Print and shaded views of the part. All mm, measured from the part's lowest x, y and z. A direction names the side the tool comes from. Round coordinates to 2 decimals unless told otherwise and drop trailing zeros. Write each loop counter-clockwise with the first axis right and the second up, starting at its lowest first coordinate (ties: lowest second). Pieces come first, ordered by that corner, then holes. Notation, with made-up numbers: (74.25, -16) - (131.25, -16) arc R7 ccw to (131.25, -5) - close; hole circle Ø3 at (-13.5, 54.25). An arc over 180 degrees is marked (long way). Put each result on its own line as item: value. Start each with the question number.
Item 1: Cut at D-D (z = 7). Give the cut face in (x, y), and give its area (3 significant figures).
Item 2: Drill centre lines: line 1 (Y direction, x = 9.5, z = 2.5); line 2 (X direction, y = 25, z = 10.5); line 3 (Z direction, x = 1, y = 16.51). Where is each one in solid material? Low to high. Write a range as from..to.
Item 3: Mould opens along X. For the marked faces 3, 4 and 5 say: released by +X, released by -X, zero draft, split by the parting line, or undercut.
Item 4: Cut at B-B (z = 2.25). Give the cut face in (x, y).
Item 5: Cut at A-A (y = 16.51). Give the cut face in (x, z).
Item 6: Pin check, flat tip, straight feed: pin 1 Ø4 at (x, y) = (11.5, 23.5) entering from -Z. Stop position of the tip, or through.
Item 7: Cut at C-C (x = 38.5). Give the cut face in (y, z).
Item 8: 3-axis set-ups, long thin cutter, end or side, ignore diameter. For the marked faces 1 and 2: which of +Z, -Z, +X, -X, +Y, -Y reach the whole face in a straight line?
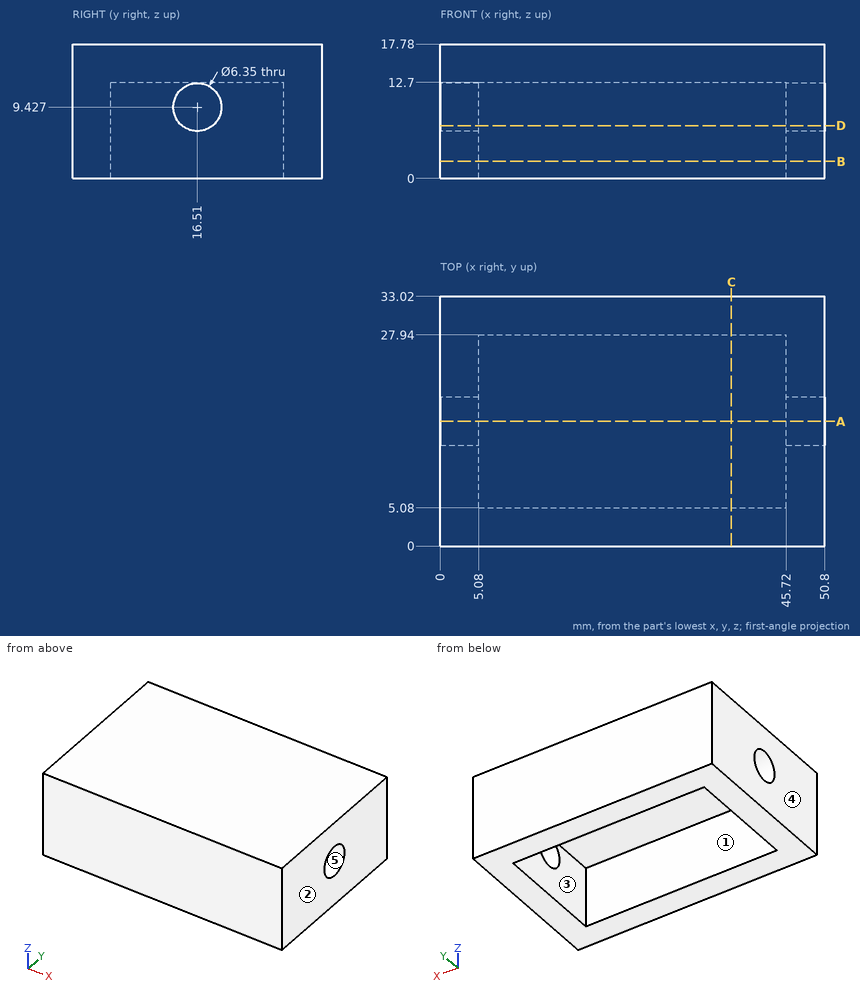
Output values:
1. outline: (0, 0) - (50.8, 0) - (50.8, 14.46) - (45.72, 14.46) - (45.72, 5.08) - (5.08, 5.08) - (5.08, 14.46) - (0, 14.46) - close; (0, 18.56) - (5.08, 18.56) - (5.08, 27.94) - (45.72, 27.94) - (45.72, 18.56) - (50.8, 18.56) - (50.8, 33.02) - (0, 33.02) - close
1. area: 707 mm2
2. line 1: 0..5.08, 27.94..33.02
2. line 2: 0..5.08, 45.72..50.8
2. line 3: 0..6.25, 12.6..17.78
3. face 3: undercut
3. face 4: released by -X
3. face 5: zero draft
4. outline: (0, 0) - (50.8, 0) - (50.8, 33.02) - (0, 33.02) - close; hole (5.08, 5.08) - (45.72, 5.08) - (45.72, 27.94) - (5.08, 27.94) - close
5. outline: (0, 0) - (5.08, 0) - (5.08, 6.25) - (0, 6.25) - close; (0, 12.6) - (5.08, 12.6) - (5.08, 12.7) - (45.72, 12.7) - (45.72, 12.6) - (50.8, 12.6) - (50.8, 17.78) - (0, 17.78) - close; (45.72, 0) - (50.8, 0) - (50.8, 6.25) - (45.72, 6.25) - close
6. pin 1: z = 12.7
7. outline: (0, 0) - (5.08, 0) - (5.08, 12.7) - (27.94, 12.7) - (27.94, 0) - (33.02, 0) - (33.02, 17.78) - (0, 17.78) - close
8. face 1: -Z
8. face 2: +Z, -Z, +X, +Y, -Y
